The model under review builds one solid part; all positions refer to its coordinate system, in mm. A direction names the side the tool comes from. Give positions to 0.01 mm unless a question says otherwise; leave off trailing zeros. Order: outer loops, then holes, each group sorted by start corner. A loop starts at its lowest first (then second) coordinate and runs counter-clockwise, first axis right, second up.
```python
from build123d import *

# Parameters (mm, degrees)
SKETCH1_R           = 1.397
BOSS_EXTRUDE1_DEPTH = 1.016
FILLET1_R           = 0.635
CUT_EXTRUDE1_DEPTH  = 0.381
CUT_EXTRUDE1_TAPER  = 5


with BuildPart() as part:
    # Sketch1 → Boss-Extrude1 (new body)
    with BuildSketch(Plane(origin=(0, 0, 0), x_dir=(1, 0, 0), z_dir=(0, 1, 0))):
        with BuildLine():
            Line((0, 0), (0, -2.54))
            Line((0, -2.54), (8.774021221, -3.97131115))
            Line((8.774021221, -3.97131115), (17.714676902, 0.85468885))
            ThreePointArc((17.714676902, 0.85468885), (21.270106923, 0.487494578), (22.230837366, -2.95531115))
            Line((22.230837366, -2.95531115), (20.32, -2.95531115))
            ThreePointArc((20.32, -2.95531115), (19.80856952, -4.601146953), (21.40873402, -5.24131115))
            ThreePointArc((21.40873402, -5.24131115), (25.94436701, -4.403774359), (30.48, -5.24131115))
            Line((30.48, -5.24131115), (37.249261314, -5.24131115))
            ThreePointArc((37.249261314, -5.24131115), (38.1, -2.06631115), (37.249261314, 1.10868885))
            Line((37.249261314, 1.10868885), (30.48, 1.10868885))
            Line((30.48, 1.10868885), (30.48, 4.91868885))
            Line((30.48, 4.91868885), (8.89, 4.91868885))
            Line((8.89, 4.91868885), (0, 0))
        make_face()
        with Locations((33.864630657, -2.06631115)):
            Circle(SKETCH1_R, mode=Mode.SUBTRACT)
    extrude(amount=BOSS_EXTRUDE1_DEPTH)

    # Fillet1
    fillet1_edges = [part.edges().sort_by_distance(p)[0] for p in [
        (30.48, 0.508, -4.91868885),
        (30.48, 0.508, -1.10868885),
        (37.249261314, 0.508, -1.10868885),
        (37.249261314, 0.508, 5.24131115),
        (20.32, 0.508, 2.95531115),
        (22.230837366, 0.508, 2.95531115),
        (0, 0.508, 2.54),
        (0, 0.508, 0),
    ]]
    fillet(fillet1_edges, radius=FILLET1_R)

    # Sketch3 → Cut-Extrude1 (cut)
    with BuildSketch(Plane(origin=(0, -0.841145333, -0.148316617), x_dir=(-1, 0, 0), z_dir=(0, -0.984807753, -0.173648178))):
        with BuildLine():
            ThreePointArc((-17.78, 3.750389462), (-13.335, 2.559355302), (-8.89, 3.750389462))
            Line((-8.89, 3.750389462), (-17.78, 3.750389462))
        make_face()
    extrude(amount=-CUT_EXTRUDE1_DEPTH, taper=CUT_EXTRUDE1_TAPER, mode=Mode.SUBTRACT)


solid = part.part
```
Item 1: Clearance check with flat-ended pins moving along their axes: pin 1 Ø2.5 at (x, z) = (33.86, 2.07) entering from +Y; pin 2 Ø0.5 at (x, y) = (32.5, 0.5) entering from +Z. State where each tip first meets the part, or that it passes through.
Values found:
pin 1: passes through
pin 2: stops at z = 5.24
Item 2: For line 1 (X direction, y = 0.2, z = 1.5); line 2 (X direction, y = 0.4, z = 1.75); line 3 (X direction, y = 0.5, z = -0.75), list the stretches that pass through material, from the lowest coordinate up.
Values found:
line 1: x = 0 to 13.35, 22.37 to 32.59, 35.14 to 38.07
line 2: x = 0 to 12.89, 22.39 to 32.5, 35.23 to 38.09
line 3: x = 1.36 to 17.52, 20.91 to 37.44
Item 3: Take a section at D-D (x = 26). Give the boundary of the cut face in (y, z).
Values found:
outline: (0, -4.92) - (1.02, -4.92) - (1.02, 4.4) - (0, 4.4) - close
Item 4: For faces 4 (the flat face through (13.182, 0.501, 1.592)), 5 (the flat face through (21.1, 0.5, 2.955)), 6 (the flat face through (30.48, 0.5, -3)), list the 3-axis set-ups (+Z, -Z, +X, -X, +Y, -Y) from which the entire face can be reached by the end or side of a thin tool; tool diameter is ignored.
Values found:
face 4: +Z, +Y, -Y
face 5: +Y, -Y
face 6: -Z, +X, +Y, -Y
Item 5: Take a section at C-C (x = 36). Give the boundary of the cut face in (y, z), and give its area (3 significant figures).
Values found:
outline: (0, -1.11) - (1.02, -1.11) - (1.02, 5.24) - (0, 5.24) - close
area: 6.45 mm2
Item 6: Take a section at A-A (z = 1.5). Give the boundary of the cut face in (x, y), and give its area (3 significant figures).
Values found:
outline: (0, 0) - (13.35, 0) - (13.35, 1.02) - (0, 1.02) - close; (22.37, 0) - (32.59, 0) - (32.59, 1.02) - (22.37, 1.02) - close; (35.14, 0) - (38.07, 0) - (38.07, 1.02) - (35.14, 1.02) - close
area: 26.9 mm2
Item 7: Take a section at B-B (y = 0.75). Give the boundary of the cut face in (x, z) (3 decimals).
Values found:
outline: (0, 0.374) arc R0.635 ccw to (0.328, -0.181) - (8.89, -4.919) - (29.845, -4.919) arc R0.635 ccw to (30.48, -4.284) - (30.48, -1.744) arc R0.635 cw to (31.115, -1.109) - (36.87, -1.109) arc R0.635 ccw to (37.438, -0.756) arc R6.35 ccw to (37.438, 4.889) arc R0.635 ccw to (36.87, 5.241) - (30.48, 5.241) arc R12.7 cw to (21.409, 5.241) arc R1.27 ccw to (20.09, 3.126) arc R0.635 ccw to (20.522, 2.955) - (21.734, 2.955) arc R0.635 cw to (22.362, 2.416) arc R3.175 cw to (17.715, -0.855) - (8.774, 3.971) - (0.533, 2.627) arc R0.635 ccw to (0, 2) - close; hole circle Ø2.794 at (33.865, 2.066)
Item 8: Draft analysis for pull direction X (two halves, no side actions). For faces 1 (the cylindrical face through (21.009, 0.501, -0.685)), 2 (the flat face through (4.7, 0.5, -2.6)), 3 (the flat face through (19, 1.016, -2)), state which applies: released by +X, released by -X, zero draft, split by the parting line, or undercut.
Values found:
face 1: undercut
face 2: released by -X
face 3: zero draft
